Autodesk Inventor part; units mm, degrees
ref_plane "YZ Plane" through (0, 0, 0) normal (1, 0, 0) x (0, 1, 0)
ref_plane "XZ Plane" through (0, 0, 0) normal (0, 1, 0) x (-1, 0, 0)
ref_plane "XY Plane" through (0, 0, 0) normal (0, 0, 1) x (1, 0, 0)
sketch "スケッチ1" plane through (0, 0, 0) normal (0, 0, 1) x (1, 0, 0)
  line L0 (-12.5, 25) -> (12.5, 25)
  line L1 (12.5, 25) -> (12.5, -25)
  line L2 (12.5, -25) -> (-12.5, -25)
  line L3 (-12.5, -25) -> (-12.5, 25)
  line L4 (-10.5, 23) -> (10.5, 23)
  line L5 (10.5, 23) -> (10.5, -23)
  line L6 (10.5, -23) -> (-10.5, -23)
  line L7 (-10.5, -23) -> (-10.5, 23)
  point P0 (0, 0)
  dimension "d0" = 25
  dimension "d1" = 50
  dimension "d2" = 46
  dimension "d3" = 21
  dimension "d4" = 25
  dimension "d5" = 23
  dimension "d6" = 10.5
  dimension "d7" = 12.5
extrude "押し出し1" add sketch "スケッチ1" along normal blind 60
sketch "スケッチ2" plane through (-12.5, 25, 0) normal (0, 1, 0) x (1, 0, 0)
  line L0 (0, 0) -> (25, 0)
  line L1 (0, 0) -> (0, -60)
  arc A0 (6, -33.5) -> (19, -33.5) centre (12.5, -33.5) ccw
  line L2 (6, -33.5) -> (6, 0)
  line L3 (19, -33.5) -> (19, 0)
  point P0 (12.5, 0)
  dimension "d10" = 13
  dimension "d11" = 33.5
  dimension "d12" = 12.5
extrude "押し出し2" cut sketch "スケッチ2" against normal blind 2
sketch "スケッチ3" plane through (-12.5, 25, 60) normal (0, 1, 0) x (1, 0, 0)
  arc A0 (6, 26.5) -> (19, 26.5) centre (12.5, 26.5) ccw
  circle A1 centre (4.5, 20) radius 1
  circle A2 centre (4.5, 56) radius 1
  circle A3 centre (20.5, 56) radius 1
  circle A4 centre (20.5, 20) radius 1
  point P0 (12.5, 60)
  dimension "d15" = 6.5
  dimension "d16" = 6.5
  dimension "d17" = 2
  dimension "d18" = 8
  dimension "d19" = 8
  dimension "d20" = 8
  dimension "d21" = 8
  dimension "d22" = 29.5
  dimension "d23" = 29.5
hole "穴1" at (-8, 25, 4) at (8, 25, 4) at (8, 25, 40) at (-8, 25, 40) direction (0, -1, 0) diameter 2 depth 2 tip angle 118 counterbore diameter 4 counterbore depth 0.5
sketch "スケッチ4" plane through (-12.5, -25, 0) normal (0, -1, 0) x (1, 0, 0)
  line L0 (25, 0) -> (0, 0)
  line L1 (25, 0) -> (25, 60)
  circle A0 centre (12.5, 10.5) radius 2
  point P0 (12.5, 0)
  dimension "d31" = 4
  dimension "d32" = 12.5
  dimension "d33" = 10.5
hole "穴2" at (0, -25, 10.5) direction (0, 1, 0) diameter 4 end through all
sketch "スケッチ5" plane through (-12.5, 25, 60) normal (0, 1, 0) x (1, 0, 0)
  line L0 (0, 0) -> (25, 0)
  arc A0 (6, 26.5) -> (19, 26.5) centre (12.5, 26.5) ccw
  circle A1 centre (20.5, 4) radius 1.5
  circle A2 centre (4.5, 4) radius 1.5
  point P0 (12.5, 60)
  dimension "d43" = 4
  dimension "d44" = 4
  dimension "d46" = 8
  dimension "d47" = 8
  dimension "d57" = 3
hole "穴4" at (-8, 25, 56) at (8, 25, 56) direction (0, -1, 0) diameter 3 end through all
thread "ねじ1"
thread "ねじ2"
thread "ねじ3"
thread "ねじ4"
sketch "スケッチ7" plane through (-12.5, -25, 0) normal (0, -1, 0) x (1, 0, 0)
  line L0 (25, 60) -> (0, 60)
  line L1 (25, 0) -> (25, 60)
  circle A0 centre (12.5, 30) radius 4
  point P0 (12.5, 0)
  dimension "d78" = 30
  dimension "d79" = 8
  dimension "d80" = 12.5
hole "穴5" at (0, -25, 30) direction (0, 1, 0) diameter 8 end through all
sketch "スケッチ8" plane through (12.5, -25, 0) normal (1, 0, 0) x (0, 0, -1)
  line L0 (-60, 50) -> (-60, 0)
  line L1 (0, 0) -> (-60, 0)
  circle A0 centre (-50, 37.5) radius 1.5
  circle A1 centre (-50, 12.5) radius 1.5
  point P0 (0, 25)
  dimension "d88" = 25
  dimension "d90" = 3
  dimension "d91" = 10
  dimension "d92" = 10
  dimension "d93" = 12.5
hole "穴6" at (12.5, -12.5, 50) at (12.5, 12.5, 50) direction (-1, 0, 0) diameter 3 end through all
properties part number "07" material "アルミニウム 6061"
Build history of the part. All positions in model axes, mm. A direction names the side the tool comes from. Round coordinates to 2 decimals unless told otherwise and drop trailing zeros. Write each loop counter-clockwise with the first axis right and the second up, starting at its lowest first coordinate (ties: lowest second). Pieces come first, ordered by that corner, then holes. Notation, with made-up numbers: (-21.75, 63) -> (3.25, 63) arc R8 cw to (3.25, 67) -> close; hole circle Ø1 at (21, -30.5). An arc over 180 degrees is marked (long way). Put each result on its own line as item: value.
Item 1: Slice it at C-C, the plane y = -8. Give the cut face in (x, z).
Here are the results:
outline: (-12.5, 0) -> (-10.5, 0) -> (-10.5, 60) -> (-12.5, 60) -> close; (10.5, 0) -> (12.5, 0) -> (12.5, 60) -> (10.5, 60) -> close
Item 2: Two-plate mould, pull along X, no slides. Class faces 1 (the face through (12.5, 0, 30)), 2 (the face through (5, -23, 30)), 3 (the face through (0, 24, 40)), 4 (the face through (-12.5, 0, 30)): pulls with the +X half, pulls with the -X half, needs draft (parallel to the pull), parting line crosses it, or undercut.
Here are the results:
face 1: pulls with the +X half
face 2: undercut
face 3: undercut
face 4: pulls with the -X half
Item 3: Slice it at B-B, the plane z = 50. Give the cut face in (x, y).
Here are the results:
outline: (-12.5, -25) -> (12.5, -25) -> (12.5, -14) -> (10.5, -14) -> (10.5, -23) -> (-10.5, -23) -> (-10.5, -14) -> (-12.5, -14) -> close; (-12.5, -11) -> (-10.5, -11) -> (-10.5, 11) -> (-12.5, 11) -> close; (-12.5, 14) -> (-10.5, 14) -> (-10.5, 23) -> (10.5, 23) -> (10.5, 14) -> (12.5, 14) -> (12.5, 25) -> (-12.5, 25) -> close; (10.5, -11) -> (12.5, -11) -> (12.5, 11) -> (10.5, 11) -> close
Item 4: Tool access for faces 5 (the face through (-6.5, 24, 17)), 6 (the face through (-7, 23, 36)), 7 (the face through (8.575, -24.014, 57.386)), 8 (the face through (-11, -2, 0)), 9 (the face through (8, 24, 41)): list every direction of +Z, -Z, +X, -X, +Y, -Y with a clear straight run to the whole face (end or side of a thin tool).
Here are the results:
face 5: -Z, +Y
face 6: +Z, -Z
face 7: +Y, -Y
face 8: -Z, +X, -X, +Y, -Y
face 9: +Y
Item 5: Slice it at A-A, the plane x = 8. Count the separate pieces of the cut face and the enclosed holes in it, plus the area to 3 significant figures.
Here are the results:
separate pieces: 6
enclosed holes: 0
area: 218 mm^2
Item 6: Flat gauge pins, fed straight in: P1, Ø6.5, axis at x = 0, z = 24.5, coming from the +Y side; P2, Ø2.5, axis at x = 8, z = 40, coming from the +Y side. Where does each tip first touch, or does it go through?
Here are the results:
P1: stops at y = -23
P2: stops at y = 24.5
Item 7: Slice it at D-D, the plane z = 10.5. Give the cut face in (x, y), plus the area to 3 significant figures.
Here are the results:
outline: (-12.5, -25) -> (-2, -25) -> (-2, -23) -> (-10.5, -23) -> (-10.5, 23) -> (-6.5, 23) -> (-6.5, 25) -> (-12.5, 25) -> close; (2, -25) -> (12.5, -25) -> (12.5, 25) -> (6.5, 25) -> (6.5, 23) -> (10.5, 23) -> (10.5, -23) -> (2, -23) -> close
area: 250 mm^2
Item 8: Wall check: probe 1 along Z at (x, y) = (-8, 23.4); probe 2 along Z at (x, y) = (-8, 24.8); probe 3 along Z at (x, y) = (0, -23.55). Give the ranges that are in metal, low to high. Write a range as from..to.
Here are the results:
probe 1: z = 0..3, 5..39, 41..54.5, 57.5..60
probe 2: z = 0..2, 6..38, 42..54.5, 57.5..60
probe 3: z = 0..8.5, 12.5..26, 34..60
